```python
from build123d import *

# Parameters (mm, degrees)
SKETCH1_W           = 110
SKETCH1_H           = 50
BOSS_EXTRUDE1_DEPTH = 40
SKETCH2_W           = 15
SKETCH2_H           = 50
CUT_EXTRUDE1_DEPTH  = 90
FILLET1_R           = 20
SKETCH3_R           = 10
CUT_EXTRUDE2_DEPTH  = 90
SKETCH4_R           = 10
BOSS_EXTRUDE2_DEPTH = 20


with BuildPart() as part:
    # Sketch1 → Boss-Extrude1 (new body)
    with BuildSketch(Plane.XY):
        Rectangle(SKETCH1_W, SKETCH1_H)
    extrude(amount=BOSS_EXTRUDE1_DEPTH)

    # Sketch2 → Cut-Extrude1 (cut)
    with BuildSketch(Plane(origin=(55, 0, 0), x_dir=(0, 0, -1), z_dir=(1, 0, 0))):
        with Locations((-20, 0)):
            Rectangle(SKETCH2_W, SKETCH2_H)
    extrude(amount=-CUT_EXTRUDE1_DEPTH, mode=Mode.SUBTRACT)

    # Fillet1
    fillet1_edges = [part.edges().sort_by_distance(p)[0] for p in [
        (55, -25, 6.25),
        (55, 25, 6.25),
        (55, -25, 33.75),
        (55, 25, 33.75),
    ]]
    fillet(fillet1_edges, radius=FILLET1_R)

    # Sketch3 → Cut-Extrude2 (cut)
    with BuildSketch(Plane.XY.offset(40)):
        with Locations((30, 0)):
            Circle(SKETCH3_R)
    extrude(amount=-CUT_EXTRUDE2_DEPTH, mode=Mode.SUBTRACT)

    # Sketch4 → Boss-Extrude2 (add)
    with BuildSketch(Plane.ZY.offset(55)):
        with Locations((20, 0)):
            Circle(SKETCH4_R)
    extrude(amount=BOSS_EXTRUDE2_DEPTH)


solid = part.part
```
Model file for the job. Use its own axes, mm. A direction names the side the tool comes from. Coordinates: 2 decimals unless noted, no trailing zeros. Write each loop counter-clockwise with the first axis right and the second up, starting at its lowest first coordinate (ties: lowest second). Pieces come first, ordered by that corner, then holes. Notation, with made-up numbers: (40, 4) - (91, 4) arc R4 cw to (91, 11) - close; hole circle Ø1 at (31, 60). An arc over 180 degrees is marked (long way). One line per item, written item: value. Start each with the question number.
1. Mould opens along Z. For faces 1 (the flat face through (-11, -25, 11)), 2 (the flat face through (11, 0, 27.5)), 3 (the flat face through (-1, 0, 40)) say: released by +Z, released by -Z, zero draft, split by the parting line, or undercut.
2. Slice it at C-C (y = 0). Write the cut outline in (x, z).
3. Slice it at A-A (x = -20.5). Write the cut outline in (y, z), plus the area to 3 significant figures.
4. Slice it at B-B (x = 30). Write the cut outline in (y, z).
5. Tool access for faces 4 (the flat face through (-1, 0, 0)), 5 (the cylindrical face through (-64.86, 3, 29.54)), 6 (the flat face through (11, 0, 12.5)): list every direction of +Z, -Z, +X, -X, +Y, -Y with a clear straight run to the whole face (end or side of a thin tool).
6. Slice it at D-D (z = 4.5). Write the cut outline in (x, y).
7. Probe line 1 (Z direction, x = 45, y = 6); line 2 (Y direction, x = 30, z = 36); line 3 (X direction, y = 19, z = 25). List the from-to ranges inside material, lowest first. Write a range as from..to.
8. Flat gauge pins, fed straight in: pin 1 (4 mm diameter, centred on y = -9, z = 16, fed in from +X); pin 2 (1 mm diameter, centred on y = -11, z = 33.5, fed in from +X); pin 3 (1 mm diameter, centred on y = -8.5, z = 29.5, fed in from +X). Where does each tip first touch, or does it go through?
Answers below:
1. face 1: zero draft
1. face 2: undercut
1. face 3: released by +Z
2. outline: (-75, 10) - (-55, 10) - (-55, 0) - (20, 0) - (20, 12.5) - (-35, 12.5) - (-35, 27.5) - (20, 27.5) - (20, 40) - (-55, 40) - (-55, 30) - (-75, 30) - close; (40, 0) - (55, 0) - (55, 12.5) - (40, 12.5) - close; (40, 27.5) - (55, 27.5) - (55, 40) - (40, 40) - close
3. outline: (-25, 0) - (25, 0) - (25, 12.5) - (-25, 12.5) - close; (-25, 27.5) - (25, 27.5) - (25, 40) - (-25, 40) - close
3. area: 1,250 mm^2
4. outline: (-25, 0) - (-10, 0) - (-10, 12.5) - (-25, 12.5) - close; (-25, 27.5) - (-10, 27.5) - (-10, 40) - (-25, 40) - close; (10, 0) - (25, 0) - (25, 12.5) - (10, 12.5) - close; (10, 27.5) - (25, 27.5) - (25, 40) - (10, 40) - close
5. face 4: -Z, +X, -X, +Y, -Y
5. face 5: -X
5. face 6: +X, +Y, -Y
6. outline: (-55, -25) - (35, -25) arc R20 ccw to (55, -5) - (55, 5) arc R20 ccw to (35, 25) - (-55, 25) - close; hole circle Ø20 at (30, 0)
7. line 1: z = 0..12.5, 27.5..40
7. line 2: y = -25..-10, 10..25
7. line 3: x = -55..-35
8. pin 1: stops at x = -35
8. pin 2: stops at x = 54.23
8. pin 3: stops at x = 54.77
